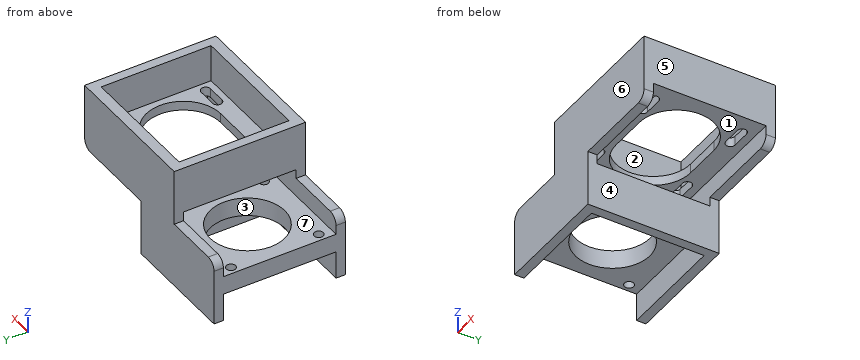
from build123d import *

# Parameters (mm, degrees)
SKETCH1_W           = 77
SKETCH1_H           = 20
SKETCH1_W_2         = 118.75
SKETCH1_H_2         = 25
SKETCH1_W_3         = 70.5
BOSS_EXTRUDE1_DEPTH = 70.5
SKETCH6_W           = 15
SKETCH6_H           = 60.5
CUT_EXTRUDE2_DEPTH  = 48.25
SKETCH7_W           = 67
SKETCH7_H           = 59
CUT_EXTRUDE3_DEPTH  = 20
CUT_EXTRUDE4_DEPTH  = 5
SKETCH9_W           = 5
SKETCH9_H           = 60.5
CUT_EXTRUDE5_DEPTH  = 48.25
SKETCH10_W          = 15
SKETCH10_H          = 60.5
CUT_EXTRUDE6_DEPTH  = 70.5
SKETCH11_W          = 5
SKETCH11_H          = 60.5
CUT_EXTRUDE7_DEPTH  = 41.75
SKETCH12_W          = 60.5
SKETCH12_H          = 60.5
CUT_EXTRUDE8_DEPTH  = 15
SKETCH13_R          = 20
SKETCH13_R_2        = 2.5
CUT_EXTRUDE9_DEPTH  = 20
SKETCH14_W          = 7.5
SKETCH14_H          = 35
SKETCH14_H_2        = 10
SKETCH14_W_2        = 34.25
SKETCH14_W_3        = 48.25
CUT_EXTRUDE10_DEPTH = 71.5
FILLET2_R           = 5


with BuildPart() as part:
    # Sketch1 → Boss-Extrude1 (new body)
    with BuildSketch(Plane(origin=(0, 0, 0), x_dir=(1, 0, 0), z_dir=(0, 1, 0))):
        with Locations((20.875, -22.5)):
            Rectangle(SKETCH1_W, SKETCH1_H)
        Rectangle(SKETCH1_W_2, SKETCH1_H_2)
        with Locations((-24.125, 22.5)):
            Rectangle(SKETCH1_W_3, SKETCH1_H)
    extrude(amount=BOSS_EXTRUDE1_DEPTH)

    # Sketch6 → Cut-Extrude2 (cut)
    with BuildSketch(Plane(origin=(59.375, 0, 0), x_dir=(0, 0, -1), z_dir=(1, 0, 0))):
        with Locations((0, 35.25)):
            Rectangle(SKETCH6_W, SKETCH6_H)
    extrude(amount=-CUT_EXTRUDE2_DEPTH, mode=Mode.SUBTRACT)

    # Sketch7 → Cut-Extrude3 (cut)
    with BuildSketch(Plane.XY.offset(32.5)):
        with Locations((20.875, 35.25)):
            Rectangle(SKETCH7_W, SKETCH7_H)
    extrude(amount=-CUT_EXTRUDE3_DEPTH, mode=Mode.SUBTRACT)

    # Sketch8 → Cut-Extrude4 (cut)
    with BuildSketch(Plane.XY.offset(12.5)):
        with BuildLine():
            Line((10.875, 55.25), (30.875, 55.25))
            ThreePointArc((30.875, 55.25), (50.875, 35.25), (30.875, 15.25))
            Line((30.875, 15.25), (10.875, 15.25))
            ThreePointArc((10.875, 15.25), (-9.125, 35.25), (10.875, 55.25))
        make_face()
        with BuildLine():
            Line((-7.695, 61.32), (2.305, 61.32))
            ThreePointArc((2.305, 61.32), (4.805, 58.82), (2.305, 56.32))
            Line((2.305, 56.32), (-7.695, 56.32))
            ThreePointArc((-7.695, 56.32), (-10.195, 58.82), (-7.695, 61.32))
        make_face()
        with BuildLine():
            Line((49.445, 61.32), (39.445, 61.32))
            ThreePointArc((39.445, 61.32), (36.945, 58.82), (39.445, 56.32))
            Line((39.445, 56.32), (49.445, 56.32))
            ThreePointArc((49.445, 56.32), (51.945, 58.82), (49.445, 61.32))
        make_face()
        with BuildLine():
            Line((-7.695, 9.18), (2.305, 9.18))
            ThreePointArc((2.305, 9.18), (4.805, 11.68), (2.305, 14.18))
            Line((2.305, 14.18), (-7.695, 14.18))
            ThreePointArc((-7.695, 14.18), (-10.195, 11.68), (-7.695, 9.18))
        make_face()
        with BuildLine():
            Line((49.445, 9.18), (39.445, 9.18))
            ThreePointArc((39.445, 9.18), (36.945, 11.68), (39.445, 14.18))
            Line((39.445, 14.18), (49.445, 14.18))
            ThreePointArc((49.445, 14.18), (51.945, 11.68), (49.445, 9.18))
        make_face()
    extrude(amount=-CUT_EXTRUDE4_DEPTH, mode=Mode.SUBTRACT)

    # Sketch9 → Cut-Extrude5 (cut)
    with BuildSketch(Plane(origin=(59.375, 0, 0), x_dir=(0, 0, -1), z_dir=(1, 0, 0))):
        with Locations((10, 35.25)):
            Rectangle(SKETCH9_W, SKETCH9_H)
    extrude(amount=-CUT_EXTRUDE5_DEPTH, mode=Mode.SUBTRACT)

    # Sketch10 → Cut-Extrude6 (cut)
    with BuildSketch(Plane.ZY.offset(59.375)):
        with Locations((0, 35.25)):
            Rectangle(SKETCH10_W, SKETCH10_H)
    extrude(amount=-CUT_EXTRUDE6_DEPTH, mode=Mode.SUBTRACT)

    # Sketch11 → Cut-Extrude7 (cut)
    with BuildSketch(Plane.ZY.offset(59.375)):
        with Locations((10, 35.25)):
            Rectangle(SKETCH11_W, SKETCH11_H)
    extrude(amount=-CUT_EXTRUDE7_DEPTH, mode=Mode.SUBTRACT)

    # Sketch12 → Cut-Extrude8 (cut)
    with BuildSketch(Plane(origin=(0, 0, -32.5), x_dir=(-1, 0, 0), z_dir=(0, 0, -1))):
        with Locations((24.125, 35.25)):
            Rectangle(SKETCH12_W, SKETCH12_H)
    extrude(amount=-CUT_EXTRUDE8_DEPTH, mode=Mode.SUBTRACT)

    # Sketch13 → Cut-Extrude9 (cut)
    with BuildSketch(Plane(origin=(0, 0, -17.5), x_dir=(-1, 0, 0), z_dir=(0, 0, -1))):
        with Locations((24.125, 35.25)):
            Circle(SKETCH13_R)
        with Locations((0.555, 58.82)):
            Circle(SKETCH13_R_2)
        with Locations((47.695, 58.82)):
            Circle(SKETCH13_R_2)
        with Locations((47.695, 11.68)):
            Circle(SKETCH13_R_2)
        with Locations((0.555, 11.68)):
            Circle(SKETCH13_R_2)
    extrude(amount=-CUT_EXTRUDE9_DEPTH, mode=Mode.SUBTRACT)

    # Sketch14 → Cut-Extrude10 (cut, through all)
    with BuildSketch(Plane(origin=(0, 70.5, 0), x_dir=(1, 0, 0), z_dir=(0, 1, 0))):
        with Locations((-55.625, 15)):
            Rectangle(SKETCH14_W, SKETCH14_H)
        with Locations((-55.625, -7.5)):
            Rectangle(SKETCH14_W, SKETCH14_H_2)
        with Locations((-34.75, -7.5)):
            Rectangle(SKETCH14_W_2, SKETCH14_H_2)
        with Locations((35.25, 7.5)):
            Rectangle(SKETCH14_W_3, SKETCH14_H_2)
    extrude(amount=-CUT_EXTRUDE10_DEPTH, mode=Mode.SUBTRACT)

    # Fillet2
    fillet2_edges = [part.edges().sort_by_distance(p)[0] for p in [
        (-51.875, 68, 2.5),
        (-51.875, 2.5, 2.5),
        (59.375, 68, -2.5),
        (59.375, 2.5, -2.5),
    ]]
    fillet(fillet2_edges, radius=FILLET2_R)


solid = part.part
Here's how the part is built. I have some questions about the finished solid (model axes, mm). Face numbers are marked on the shaded views. A direction names the side the tool comes from. Coordinates: 2 decimals unless noted, no trailing zeros. Loops run counter-clockwise (first coordinate to the right, second up) from the corner with the lowest first, then second, coordinate; pieces in that order, holes last.
1. For P1, Ø16.5, axis at x = 23.5, z = -0.5, coming from the -Y side; P2, Ø5.5, axis at x = 26.5, y = 3, coming from the -Z side; P3, Ø16, axis at y = 29, z = 19.5, coming from the -X side (3 decimals); P4, Ø3, axis at x = 5, y = 8, coming from the +Z side, each with a flat end and sliding along its axis, tell me the tip position at first contact or that it passes through.
2. Imagine slicing it at D-D, the plane z = -25.5. Please give me the cut outline in (x, y) (3 decimals), and give its area (4 significant figures).
3. Imagine slicing it at B-B, the plane y = 35.25. Please give me the cut outline in (x, z) (3 decimals).
4. Imagine slicing it at C-C, the plane y = 58.82. Count the separate pieces of the cut face and the enclosed holes in it, and give its area (3 significant figures).
5. If we mould it in two halves opening along Y, with no side actions, what happens to the marked faces 5, 6 and 7? For each: pulls with the +Y half, pulls with the -Y half, needs draft (parallel to the pull), parting line crosses it, or undercut.
6. For the marked faces 1, 2, 3 and 4, which set-ups out of +Z, -Z, +X, -X, +Y, -Y let a thin tool reach every point of the face, with its end or its side?
7. I need wall thicknesses on L1, parallel to Y at x = -23.5, z = 0; L2, parallel to Y at x = 52.5, z = 21.5; L3, parallel to X at y = 49.5, z = 14 (3 decimals). Which ranges of each line are inside material? Lowest first, please.
8. Imagine slicing it at A-A, the plane z = 15. Please give me the cut outline in (x, y) (3 decimals).
Taken from the geometry:
1. P1: stops at y = 0
1. P2: stops at z = -2.5
1. P3: stops at x = -17.625
1. P4: stops at z = 12.5
2. outline: (-51.875, 0) - (11.125, 0) - (11.125, 70.5) - (-51.875, 70.5) - (-51.875, 65.5) - (6.125, 65.5) - (6.125, 5) - (-51.875, 5) - close
2. area: 932.5 mm2
3. outline: (-51.875, -17.5) - (-44.125, -17.5) - (-44.125, -7.5) - (-51.875, -7.5) - close; (-17.625, 7.5) - (-9.125, 7.5) - (-9.125, 12.5) - (-12.625, 12.5) - (-12.625, 32.5) - (-17.625, 32.5) - close; (-4.125, -17.5) - (6.125, -17.5) - (6.125, -32.5) - (11.125, -32.5) - (11.125, -7.5) - (-4.125, -7.5) - close; (50.875, 7.5) - (59.375, 7.5) - (59.375, 32.5) - (54.375, 32.5) - (54.375, 12.5) - (50.875, 12.5) - close
4. separate pieces: 6
4. enclosed holes: 0
4. area: 1,040 mm2
5. face 5: needs draft
5. face 6: pulls with the -Y half
5. face 7: undercut
6. face 1: +X, -X
6. face 2: +Z
6. face 3: -Z
6. face 4: -Z, +X, +Y, -Y
7. L1: y = 0 to 5, 65.5 to 70.5
7. L2: y = 0 to 5.75, 64.75 to 70.5
7. L3: x = -17.625 to -12.625, 54.375 to 59.375
8. outline: (-17.625, 0) - (59.375, 0) - (59.375, 70.5) - (-17.625, 70.5) - close; hole (-12.625, 5.75) - (54.375, 5.75) - (54.375, 64.75) - (-12.625, 64.75) - close
